Design review of the part built by this model. Coordinates are the model's own, in mm. A direction names the side the tool comes from. Round coordinates to 2 decimals unless told otherwise and drop trailing zeros. Loops run counter-clockwise (first coordinate to the right, second up) from the corner with the lowest first, then second, coordinate; pieces in that order, holes last. Notation, with made-up numbers: (-36.5, 48) - (12.5, 48) arc R28 ccw to (12.5, 86) - close; hole circle Ø5 at (16, 28.5). An arc over 180 degrees is marked (long way). Use one line per item in the form item = value. Start each with the question number.
(1) Wall thickness on probe 1 along Z at (x, y) = (-15.5, 38.5) (3 decimals); probe 2 along Z at (x, y) = (-1.5, 61): over which ranges is each line inside the solid? List them lowest first. Write a range as [from, to].
(2) We need section B-B, the plane x = -70. Write out the cut boundary in (y, z) (1 decimal), then the cut area to 3 significant figures.
(3) The part is to be moulded in two halves that separate along X. For faces 6 (the flat face through (109.538, 65, -2)), 7 (the flat face through (-103.188, 65, 1)), 8 (the flat face through (-109.538, 65, 2)), 9 (the flat face through (1, 65, 103.188)), say which applies: released by +X, released by -X, zero draft, split by the parting line, or undercut.
(4) We need section C-C, the plane y = 66. Write out the cut boundary in (x, z).
(5) We need section D-D, the plane y = 37. Write out the cut boundary in (x, z) (1 decimal), then the cut area to 3 significant figures.
(6) We need section A-A, the plane z = -58.5. Write out the cut boundary in (x, y) (1 decimal), then the cut area to 3 significant figures.
(7) Machinability: for faces 1 (the flat face through (-103.188, 29, 1)), 2 (the flat face through (-1, 29, -101.6)), 3 (the flat face through (1, 29, 101.6)), 4 (the flat face through (-99, 60.325, 0)), 5 (the flat face through (-9, 70.485, 105)), which of the approach directions +Z, -Z, +X, -X, +Y, -Y give a long, thin tool a straight path to every point of the face, cutting with its end or side? Answer none if there is none.
(8) For pin 1 (1 mm diameter, centred on y = 29.5, z = -73.5, fed in from +X) (3 decimals); pin 2 (18 mm diameter, centred on x = 6, y = 21.5, fed in from +Z); pin 3 (3.5 mm diameter, centred on y = 39.5, z = -100, fed in from +X), all flat-tipped, find the tip position at first contact; note any pin that passes through.
Autodesk Inventor part; units mm, degrees
ref_plane "Work Plane1" through (0, 58.7375, 0) normal (0, 1, 0) x (1, 0, 0)
ref_plane "YZ Plane" through (0, 0, 0) normal (1, 0, 0) x (0, 1, 0)
ref_plane "XZ Plane" through (0, 0, 0) normal (0, 1, 0) x (-1, 0, 0)
sketch "Sketch1" plane through (0, 0, 0) normal (0, 1, 0) x (-1, 0, 0)
  line L0 (-103.1875, 101.6) -> (103.1875, 101.6)
  line L1 (103.1875, 101.6) -> (103.1875, -101.6)
  line L2 (103.1875, -101.6) -> (-103.1875, -101.6)
  line L3 (-103.1875, -101.6) -> (-103.1875, 101.6)
  line L4 (-103.1875, 101.6) -> (103.1875, -101.6) construction
  line L5 (103.1875, 101.6) -> (-103.1875, -101.6) construction
  line L6 (-98.425, 98.425) -> (98.425, 98.425)
  line L7 (98.425, 98.425) -> (98.425, -98.425)
  line L8 (98.425, -98.425) -> (-98.425, -98.425)
  line L9 (-98.425, -98.425) -> (-98.425, 98.425)
  line L10 (-98.425, 98.425) -> (98.425, -98.425) construction
  line L11 (98.425, 98.425) -> (-98.425, -98.425) construction
  point P0 (0, 0)
  dimension "d0" = 203.2
  dimension "d1" = 206.375
  dimension "d2" = 196.85
extrude "Extrusion1" add sketch "Sketch1" along normal blind 60.325
ref_plane "Work Plane1" through (0, 58.7375, 0) normal (0, 1, 0) x (1, 0, 0)
sketch "Sketch2" plane through (0, 58.7375, 0) normal (0, 1, 0) x (1, 0, 0)
  line L0 (109.5375, -109.5375) -> (-109.5375, -109.5375)
  line L1 (-109.5375, -109.5375) -> (-109.5375, 109.5375)
  line L2 (-109.5375, 109.5375) -> (109.5375, 109.5375)
  line L3 (109.5375, 109.5375) -> (109.5375, -109.5375)
  line L4 (109.5375, -109.5375) -> (-109.5375, 109.5375) construction
  line L5 (-109.5375, -109.5375) -> (109.5375, 109.5375) construction
  line L6 (103.1875, 101.6) -> (-103.1875, 101.6)
  line L7 (-103.1875, 101.6) -> (-103.1875, -101.6)
  line L8 (-103.1875, -101.6) -> (103.1875, -101.6)
  line L9 (103.1875, -101.6) -> (103.1875, 101.6)
  line L10 (98.425, -98.425) -> (-98.425, -98.425)
  line L11 (-98.425, -98.425) -> (-98.425, 98.425)
  line L12 (-98.425, 98.425) -> (98.425, 98.425)
  line L13 (98.425, 98.425) -> (98.425, -98.425)
  point P0 (0, 0)
  dimension "d7" = 219.075
extrude "Extrusion2" add sketch "Sketch2" along normal up to surface (1.5875 mm away) contours L0 L1 L2 L3
sketch "Sketch3" plane through (0, 60.325, 0) normal (0, 1, 0) x (1, 0, 0)
  line L0 (109.5375, 109.5375) -> (109.5375, -109.5375)
  line L1 (-109.5375, 109.5375) -> (109.5375, 109.5375)
  line L2 (-109.5375, -109.5375) -> (-109.5375, 109.5375)
  line L3 (109.5375, -109.5375) -> (-109.5375, -109.5375)
  line L4 (98.425, -98.425) -> (-98.425, -98.425)
  line L5 (-98.425, -98.425) -> (-98.425, 98.425)
  line L6 (-98.425, 98.425) -> (98.425, 98.425)
  line L7 (98.425, 98.425) -> (98.425, -98.425)
  line L8 (103.1875, -103.1875) -> (-103.1875, -103.1875)
  line L9 (-103.1875, -103.1875) -> (-103.1875, 103.1875)
  line L10 (-103.1875, 103.1875) -> (103.1875, 103.1875)
  line L11 (103.1875, 103.1875) -> (103.1875, -103.1875)
  line L12 (103.1875, -103.1875) -> (-103.1875, 103.1875) construction
  line L13 (-103.1875, -103.1875) -> (103.1875, 103.1875) construction
  point P0 (0, 0)
  dimension "d10" = 206.375
extrude "Extrusion3" add sketch "Sketch3" along normal blind 10.16 contours L0 L3 L2 L1
sketch "Sketch4" plane through (103.1875, 0, 101.6) normal (1, 0, 0) x (0, 0, -1)
  line L0 (200.025, 0) -> (3.175, 0)
  line L1 (3.175, 0) -> (3.175, 60.325)
  line L2 (200.025, 60.325) -> (3.175, 60.325)
  line L3 (200.025, 0) -> (200.025, 60.325)
  point P0 (101.6, 0)
extrude "Extrusion4" cut sketch "Sketch4" against normal blind 10.16
properties part number "wall support"
Data:
q1.probe_1 = [-101.6, -98.425], [98.425, 101.6]
q1.probe_2 = [-109.54, -103.19], [103.19, 109.54]
q2.outline = (0, -101.6) - (58.7, -101.6) - (58.7, -109.5) - (70.5, -109.5) - (70.5, -103.2) - (60.3, -103.2) - (60.3, -98.4) - (0, -98.4) - close; (0, 98.4) - (60.3, 98.4) - (60.3, 103.2) - (70.5, 103.2) - (70.5, 109.5) - (58.7, 109.5) - (58.7, 101.6) - (0, 101.6) - close
q2.area = 537 mm^2
q3.face_6 = released by +X
q3.face_7 = undercut
q3.face_8 = released by -X
q3.face_9 = undercut
q4.outline = (-109.54, -109.54) - (109.54, -109.54) - (109.54, 109.54) - (-109.54, 109.54) - close; hole (-103.19, -103.19) - (103.19, -103.19) - (103.19, 103.19) - (-103.19, 103.19) - close
q5.outline = (-103.2, -101.6) - (103.2, -101.6) - (103.2, -98.4) - (-98.4, -98.4) - (-98.4, 98.4) - (103.2, 98.4) - (103.2, 101.6) - (-103.2, 101.6) - close
q5.area = 2,250 mm^2
q6.outline = (-109.5, 58.7) - (-103.2, 58.7) - (-103.2, 0) - (-98.4, 0) - (-98.4, 60.3) - (-103.2, 60.3) - (-103.2, 70.5) - (-109.5, 70.5) - close; (103.2, 58.7) - (109.5, 58.7) - (109.5, 70.5) - (103.2, 70.5) - close
q6.area = 436 mm^2
q7.face_1 = +Z, -Z, -X, -Y
q7.face_2 = -Z, +X, -X, -Y
q7.face_3 = +Z, +X, -X, -Y
q7.face_4 = +Y
q7.face_5 = +Z, -Z, +X, -X, +Y
q8.pin_1 = -98.425
q8.pin_2 = 101.6
q8.pin_3 = 103.19
